Design review of the part shown in the three views and the two pictorial views. Dimensions are in mm from the part's minimum x, y and z. Coordinates: 2 decimals unless noted, no trailing zeros. Order: outer loops, then holes, each group sorted by start corner. A loop starts at its lowest first (then second) coordinate and runs counter-clockwise, first axis right, second up. Notation, with made-up numbers: (27.25, 41.25) -> (33.25, 41.25) arc R25 cw to (33.25, 77.25) -> close; hole circle Ø4 at (-37, -37). An arc over 180 degrees is marked (long way). Answer as a JSON object with one key per item and string values. Group by question number.
1) Add section A-A, the plane y = 23. Write out the cut boundary in (x, z).
2) Add section B-B, the plane z = 45. Write out the cut boundary in (x, y), then the cut area to 3 significant figures.
3) For pin 1 (0.9 mm diameter, centred on x = 1.5, z = 4.5, fed in from -Y); pin 2 (1.5 mm diameter, centred on x = 1.5, z = 88, fed in from +Y); pin 3 (1.5 mm diameter, centred on x = 1, y = 2, fed in from +Z); pin 4 (6 mm diameter, centred on y = 10, z = 74, fed in from -X), all flat-tipped, find the tip position at first contact; note any pin that passes through.
4) Wall thickness on L1, parallel to Z at x = 0.95, y = 23.5; L2, parallel to Y at x = 0.6, z = 6: over which ranges is each line inside the solid? List them lowest first.
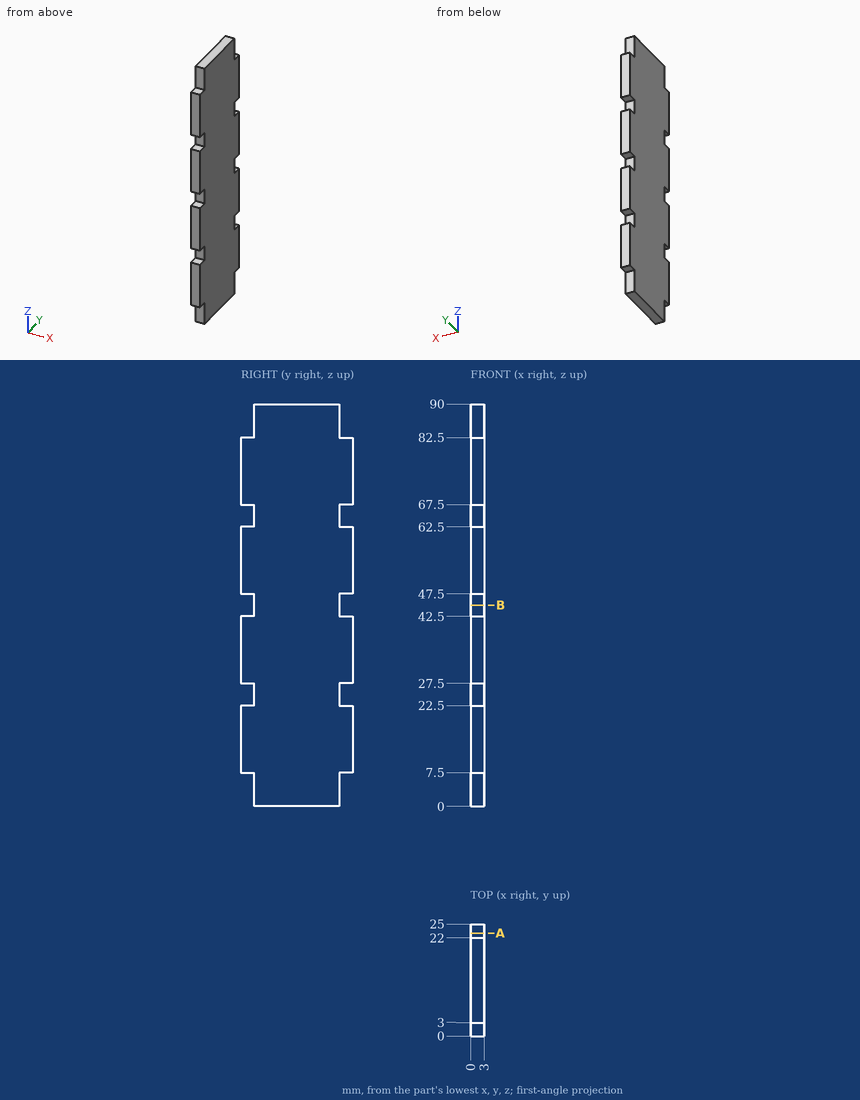
Output values:
{
 "1": {"outline": "(0, 7.5) -> (3, 7.5) -> (3, 22.5) -> (0, 22.5) -> close; (0, 27.5) -> (3, 27.5) -> (3, 42.5) -> (0, 42.5) -> close; (0, 47.5) -> (3, 47.5) -> (3, 62.5) -> (0, 62.5) -> close; (0, 67.5) -> (3, 67.5) -> (3, 82.5) -> (0, 82.5) -> close"},
 "2": {"outline": "(0, 3) -> (3, 3) -> (3, 22) -> (0, 22) -> close", "area": "57.0 mm²"},
 "3": {"pin 1": "stops at y = 3", "pin 2": "stops at y = 22", "pin 3": "stops at z = 82.5", "pin 4": "stops at x = 0"},
 "4": {"L1": "z = 7.5 to 22.5, 27.5 to 42.5, 47.5 to 62.5, 67.5 to 82.5", "L2": "y = 3 to 22"}
}
